```python
from build123d import *

# Parameters (mm, degrees)
ESQUISSE1_W             = 31
ESQUISSE1_H             = 23.85
BOSS_EXTRU_1_DEPTH      = 3.2
ESQUISSE2_W             = 26.7
ESQUISSE2_H             = 19.8
BOSS_EXTRU_2_DEPTH      = 20.3
ESQUISSE3_W             = 24
ESQUISSE3_H             = 16
ENL_V_MAT_EXTRU_1_DEPTH = 17
CHANFREIN1_SIZE         = 5
BOSS_EXTRU_3_DEPTH      = 16
BOSS_EXTRU_3_DEPTH_BACK = 12
ESQUISSE4_W             = 1.5
ESQUISSE4_H             = 6.3
CONG_1_R                = 2
CONG_2_R                = 0.5


with BuildPart() as part:
    # Esquisse1 → Boss.-Extru.1 (new body)
    with BuildSketch(Plane.XY):
        Rectangle(ESQUISSE1_W, ESQUISSE1_H)
    extrude(amount=BOSS_EXTRU_1_DEPTH)

    # Esquisse2 → Boss.-Extru.2 (add)
    with BuildSketch(Plane(origin=(0, 0, 0), x_dir=(-1, 0, 0), z_dir=(0, 0, -1))):
        Rectangle(ESQUISSE2_W, ESQUISSE2_H)
    extrude(amount=-BOSS_EXTRU_2_DEPTH)

    # Esquisse3 → Enlèv. mat.-Extru.1 (cut)
    with BuildSketch(Plane(origin=(0, 0, 0), x_dir=(-1, 0, 0), z_dir=(0, 0, -1))):
        Rectangle(ESQUISSE3_W, ESQUISSE3_H)
    extrude(amount=-ENL_V_MAT_EXTRU_1_DEPTH, mode=Mode.SUBTRACT)

    # Chanfrein1
    chanfrein1_edges = [part.edges().sort_by_distance(p)[0] for p in [
        (-12, 8, 8.5),
        (12, 8, 8.5),
    ]]
    chamfer(chanfrein1_edges, length=CHANFREIN1_SIZE)

    # Esquisse4 → Boss.-Extru.3 (add, two sides: drawn at the far end of the back side and taken through both)
    with BuildSketch(Plane(origin=(0, 0, 17), x_dir=(-1, 0, 0), z_dir=(0, 0, -1)).offset(-BOSS_EXTRU_3_DEPTH_BACK)):
        with Locations((0, 3.85)):
            Rectangle(ESQUISSE4_W, ESQUISSE4_H)
        with Locations((-7.5, -3.85)):
            Rectangle(ESQUISSE4_W, ESQUISSE4_H)
        with Locations((7.5, -3.85)):
            Rectangle(ESQUISSE4_W, ESQUISSE4_H)
    extrude(amount=BOSS_EXTRU_3_DEPTH + BOSS_EXTRU_3_DEPTH_BACK)

    # Congé1
    cong_1_edges = [part.edges().sort_by_distance(p)[0] for p in [
        (-13.35, 9.9, 11.75),
        (-13.35, -9.9, 11.75),
        (13.35, -9.9, 11.75),
        (13.35, 9.9, 11.75),
        (-12, -8, 8.5),
        (12, -8, 8.5),
        (12, 3, 8.5),
        (-7, 8, 8.5),
        (7, 8, 8.5),
        (-12, 3, 8.5),
        (15.5, -11.925, 1.6),
        (-15.5, -11.925, 1.6),
        (-15.5, 11.925, 1.6),
        (15.5, 11.925, 1.6),
    ]]
    fillet(cong_1_edges, radius=CONG_1_R)

    # Congé2
    cong_2_edges = [part.edges().sort_by_distance(p)[0] for p in [
        (-6.75, -3.85, 20.3),
        (-7.5, -7, 20.3),
        (-8.25, -3.85, 20.3),
        (15.5, 0, 0),
        (0, 8, 0),
        (-9.5, 5.5, 0),
        (-12, -1.914213562, 0),
        (0, -8, 0),
        (12, -1.914213562, 0),
        (9.5, 5.5, 0),
        (0, -11.925, 0),
        (-15.5, 0, 0),
        (0, 11.925, 0),
        (14.914213562, 11.339213562, 0),
        (-14.914213562, 11.339213562, 0),
        (-14.914213562, -11.339213562, 0),
        (14.914213562, -11.339213562, 0),
        (13.35, 0, 20.3),
        (0, -9.9, 20.3),
        (-13.35, 0, 20.3),
        (0, 9.9, 20.3),
        (12.764213562, 9.314213562, 20.3),
        (-12.764213562, 9.314213562, 20.3),
        (-12.764213562, -9.314213562, 20.3),
        (12.764213562, -9.314213562, 20.3),
        (-11.414213562, -7.414213562, 0),
        (-11.847759065, 2.93693974, 0),
        (-6.93693974, 7.847759065, 0),
        (6.93693974, 7.847759065, 0),
        (11.414213562, -7.414213562, 0),
        (11.847759065, 2.93693974, 0),
        (0, 7, 20.3),
        (0.75, 3.85, 20.3),
        (0, 0.7, 20.3),
        (-0.75, 3.85, 20.3),
        (7.5, -0.7, 20.3),
        (8.25, -3.85, 20.3),
        (7.5, -7, 20.3),
        (6.75, -3.85, 20.3),
        (-7.5, -0.7, 20.3),
    ]]
    fillet(cong_2_edges, radius=CONG_2_R)


solid = part.part
```
For this review, take the finished solid that the model builds, in its own axes (mm). A direction names the side the tool comes from. Give positions to 0.01 mm unless a question says otherwise; leave off trailing zeros. Loops run counter-clockwise (first coordinate to the right, second up) from the corner with the lowest first, then second, coordinate; pieces in that order, holes last. Notation, with made-up numbers: M 46,9 L 88,9 A11 ccw 88,26 Z; hole C 15,22 d7. An arc over 180 degrees is marked long. One line per item, written item: value. Start each with the question number.
Q1. Add section B-B (x = 5). Give the boundary of the cut face in (y, z) (3 decimals), and give its area (3 significant figures).
Q2. Add section A-A (z = 14.75). Count the separate pieces of the cut face and the enclosed holes in it, and give its area (3 significant figures).
Q3. Draft analysis for pull direction Y (two halves, no side actions). For faces 1 (the face through (-11.85, 2.93, 8.87)), 2 (the face through (-7, -7, 25)), 3 (the face through (-15.5, 0, 2)), state which applies: released by +Y, released by -Y, zero draft, split by the parting line, or undercut.
Q4. Machinability: for faces 4 (the face through (0, -11.925, 2)), 5 (the face through (-13.35, 0, 11)), 6 (the face through (-9.633, 5.58, 0.143)), 7 (the face through (0, -9.9, 11)), 8 (the face through (6.75, -4, 25)), which of the approach directions +Z, -Z, +X, -X, +Y, -Y give a long, thin tool a straight path to every point of the face, cutting with its end or side? Answer none if there is none.
Q5. Add section C-C (z = 22.5). Give the boundary of the cut face in (x, y).
Q6. For L1, parallel to X at y = -5.25, z = 12.5; L2, parallel to Y at x = 0.5, z = 2 (3 decimals); L3, parallel to X at y = 6, z = 27.25, list the stretches that pass through material, from the lowest coordinate up.
Q7. Add section D-D (z = 18.5). Give the boundary of the cut face in (x, y), and give its area (3 significant figures).
Q8. Clearance check with flat-ended pins moving along their axes: pin 1 Ø1 at (x, z) = (8, 22) entering from -Y; pin 2 Ø2 at (x, z) = (-10.5, 14.5) entering from +Y; pin 3 Ø3 at (y, z) = (5, 25.5) entering from +X. State where each tip first meets the part, or that it passes through.
Reply:
1. outline: M -11.925,0.5 A0.5 ccw -11.425,0 L -8.5,0 A0.5 ccw -8,0.5 L -8,17 L 8,17 L 8,0.5 A0.5 ccw 8.5,0 L 11.425,0 A0.5 ccw 11.925,0.5 L 11.925,3.2 L 9.9,3.2 L 9.9,19.8 A0.5 ccw 9.4,20.3 L -9.4,20.3 A0.5 ccw -9.9,19.8 L -9.9,3.2 L -11.925,3.2 Z
1. area: 143 mm²
2. separate pieces: 4
2. enclosed holes: 1
2. area: 197 mm²
3. face 1: undercut
3. face 2: released by -Y
3. face 3: zero draft
4. face 4: +Z, -Z, +X, -X, -Y
4. face 5: +Z, -X, +Y, -Y
4. face 6: -Z
4. face 7: +Z, +X, -X, -Y
4. face 8: +Z, +Y, -Y
5. outline: M -8.25,-7 L -6.75,-7 L -6.75,-0.7 L -8.25,-0.7 Z; M -0.75,0.7 L 0.75,0.7 L 0.75,7 L -0.75,7 Z; M 6.75,-7 L 8.25,-7 L 8.25,-0.7 L 6.75,-0.7 Z
6. L1: -13.35 to -12, -8.25 to -6.75, 6.75 to 8.25, 12 to 13.35
6. L2: -11.925 to -8, 0.7 to 7, 8 to 11.925
6. L3: -0.75 to 0.75
7. outline: M -13.35,-7.9 A2 ccw -11.35,-9.9 L 11.35,-9.9 A2 ccw 13.35,-7.9 L 13.35,7.9 A2 ccw 11.35,9.9 L -11.35,9.9 A2 ccw -13.35,7.9 Z
7. area: 525 mm²
8. pin 1: y = -7
8. pin 2: y = 9.9
8. pin 3: x = 0.75
